Autodesk Inventor part; units mm, degrees
ref_plane "YZ Plane" through (0, 0, 0) normal (1, 0, 0) x (0, 1, 0)
ref_plane "XZ Plane" through (0, 0, 0) normal (0, 1, 0) x (-1, 0, 0)
ref_plane "XY Plane" through (0, 0, 0) normal (0, 0, 1) x (1, 0, 0)
sketch "Sketch1" plane through (0, 0, 0) normal (0, 1, 0) x (-1, 0, 0)
  circle A0 centre (0, 0) radius 3.5
  line L0 (0, -5) -> (-40, -5)
  line L1 (-40, -5) -> (-40, 5) construction
  line L2 (-40, 5) -> (0, 5)
  line L3 (0, 5) -> (0, -5) construction
  line L4 (-74, -8.5) -> (-40, -8.5)
  line L5 (-40, -8.5) -> (-40, 8.5)
  line L6 (-40, 8.5) -> (-74, 8.5)
  line L7 (-74, 8.5) -> (-74, -8.5)
  line L8 (20.8, 0) -> (-89.8, 0)
  line L9 (0, -11.9) -> (0, 11.9)
  arc A1 (0, -5) -> (0, 5) centre (0, 0) ccw
  line L10 (0, 0) -> (0, -5) construction
  line L11 (0, 0) -> (5, 0) construction
  line L12 (0, 0) -> (0, 5) construction
  line L13 (-57, -8.5) -> (-57, 8.5) construction
  line L14 (-45, -6.25) -> (-69, -6.25)
  line L15 (-69, -6.25) -> (-69, 6.25)
  line L16 (-69, 6.25) -> (-45, 6.25)
  line L17 (-45, 6.25) -> (-45, -6.25)
  line L18 (-45, -6.25) -> (-69, 6.25) construction
  line L19 (-69, -6.25) -> (-45, 6.25) construction
  line L20 (-43.25, 0) -> (-70.75, 0) construction
  circle A2 centre (-43.25, 0) radius 1
  circle A3 centre (-70.75, 0) radius 1
  point P0 (-40, 0)
  point P1 (-57, 0)
  point P2 (-57, 0)
  dimension "d0" = 7
  dimension "d2" = 5
  dimension "d3" = 90
  dimension "d4" = 180
  dimension "d5" = 24
  dimension "d6" = 12.5
  dimension "d7" = 17
  dimension "d8" = 34
  dimension "d9" = 2
  dimension "d10" = 27.5
  dimension "d11" = 40
extrude "Extrusion1" add sketch "Sketch1" along normal blind 5 contours L8 A1 L9 A0 | A0 L9 A1 L8 | A0 L8 L5 L2 L9 | L9 L0 L5 L8 A0 | L8 A2 L17 L16 L15 A3 L7 L6 L5 | L5 L4 L7 L8 A3 L15 L14 L17 A2
sketch "Sketch2" plane through (0, 5, 0) normal (0, 1, 0) x (1, 0, 0)
  circle A0 centre (0, 0) radius 3
  arc A1 (14, -2) -> (14, 2) centre (14, 0) ccw
  line L0 (14, 0) -> (14, 2) construction
  line L1 (14, 0) -> (16, 0) construction
  line L2 (14, 0) -> (14, -2) construction
  line L3 (0, 11.9) -> (0, -11.9)
  line L4 (-20.8, 0) -> (89.8, 0)
  line L5 (14, 2) -> (0, 3)
  line L6 (14, -2) -> (0, -3)
  dimension "d14" = 6
  dimension "d16" = 90
  dimension "d17" = 180
  dimension "d18" = 14
  dimension "d22" = 2
extrude "Extrusion2" cut sketch "Sketch2" against normal blind 2.5 contours L4 L3 L5 A0 | L4 A1 L6 A0 | A0 L6 L3 L4 | A0 L5 A1 L4 | L4 A0 L3 | L3 A0 L4
fillet "Fillet1" radius 2 6 edges at (40, 2.5, 8.5) (74, 2.5, 8.5) (74, 2.5, -8.5) (40, 2.5, -8.5) (40, 2.5, -5) (40, 2.5, 5)
properties part number "link2"
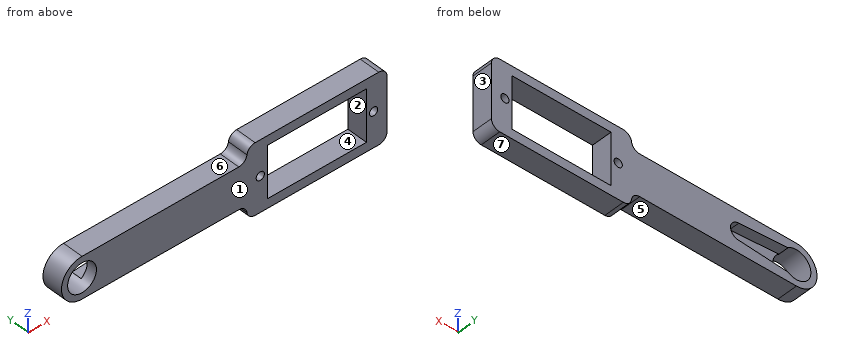
Build history of the part. All positions in model axes, mm. Face numbers are marked on the shaded views. A direction names the side the tool comes from. Round coordinates to 2 decimals unless told otherwise and drop trailing zeros. Write each loop counter-clockwise with the first axis right and the second up, starting at its lowest first coordinate (ties: lowest second). Pieces come first, ordered by that corner, then holes. Notation, with made-up numbers: (50, 45.5) - (71, 45.5) arc R25 cw to (71, 76.5) - close; hole circle Ø2 at (-10, 78). An arc over 180 degrees is marked (long way). Answer as CSV lines item,"result".
Q1. Pull direction X, two halves, no side cores. Call the marked faces 1, 2 and 3: +X half, -X half, draft (parallel to the pull), parting line (faces both ways), or undercut.
Report:
face 1,"draft"
face 2,"undercut"
face 3,"+X half"
Q2. Cut at B-B (x = 43.25). Write the cut outline in (y, z).
Report:
outline,"(0, -8.5) - (5, -8.5) - (5, -1) - (0, -1) - close; (0, 1) - (5, 1) - (5, 8.5) - (0, 8.5) - close"
Q3. Drop flat-ended pins along their axis: pin 1 (1.5 mm diameter, centred on x = 20.5, y = 3.5, fed in from -Z); pin 2 (1.5 mm diameter, centred on x = 14, y = 3, fed in from +Z); pin 3 (1.7 mm diameter, centred on x = 11, z = -1, fed in from +Y); pin 4 (5.5 mm diameter, centred on x = 0, z = 0, fed in from +Y). Give the stop position or say it passes through.
Report:
pin 1,"stops at z = -5"
pin 2,"stops at z = 5"
pin 3,"stops at y = 2.5"
pin 4,"passes through"
Q4. Cut at C-C (x = 65). Write the cut outline in (y, z).
Report:
outline,"(0, -8.5) - (5, -8.5) - (5, -6.25) - (0, -6.25) - close; (0, 6.25) - (5, 6.25) - (5, 8.5) - (0, 8.5) - close"
Q5. Cut at D-D (y = 1.4). State how many separate pieces and enclosed holes the cut face has, and give its area (3 significant figures).
Report:
separate pieces,"1"
enclosed holes,"4"
area,"671 mm^2"
Q6. Cut at A-A (z = 0). Write the cut outline in (x, y).
Report:
outline,"(-5, 0) - (-3.5, 0) - (-3.5, 5) - (-5, 5) - close; (3.5, 0) - (42.25, 0) - (42.25, 5) - (16, 5) - (16, 2.5) - (3.5, 2.5) - close; (44.25, 0) - (45, 0) - (45, 5) - (44.25, 5) - close; (69, 0) - (69.75, 0) - (69.75, 5) - (69, 5) - close; (71.75, 0) - (74, 0) - (74, 5) - (71.75, 5) - close"
Q7. Tool access for the marked faces 4, 5, 6 and 7: list every direction of +Z, -Z, +X, -X, +Y, -Y with a clear straight run to the whole face (end or side of a thin tool).
Report:
face 4,"+Y, -Y"
face 5,"-Z, -X, +Y, -Y"
face 6,"+Z, -X, +Y, -Y"
face 7,"-Z, +X, -X, +Y, -Y"
Q8. Drill centre lines: probe 1 along X at (y, z) = (2.1, 0); probe 2 along X at (y, z) = (3.4, 0); probe 3 along Z at (x, y) = (48, 1.5). Where is each one in solid material? Low to high. Write a range as [from, to].
Report:
probe 1,"x = [-5, -3.5], [3.5, 42.25], [44.25, 45], [69, 69.75], [71.75, 74]"
probe 2,"x = [-5, -3.5], [16, 42.25], [44.25, 45], [69, 69.75], [71.75, 74]"
probe 3,"z = [-8.5, -6.25], [6.25, 8.5]"
